CAD build for the part. Positions are in the model's coordinates, mm. Face numbers are marked on the shaded views. A direction names the side the tool comes from. Coordinates: 2 decimals unless noted, no trailing zeros. Order: outer loops, then holes, each group sorted by start corner. A loop starts at its lowest first (then second) coordinate and runs counter-clockwise, first axis right, second up. Notation, with made-up numbers: (68.25, -9.5) - (105.25, -9.5) arc R26 ccw to (105.25, 16.5) - close; hole circle Ø9 at (43.25, -5.5). An arc over 180 degrees is marked (long way). Return JSON: item names as keys, results as strings.
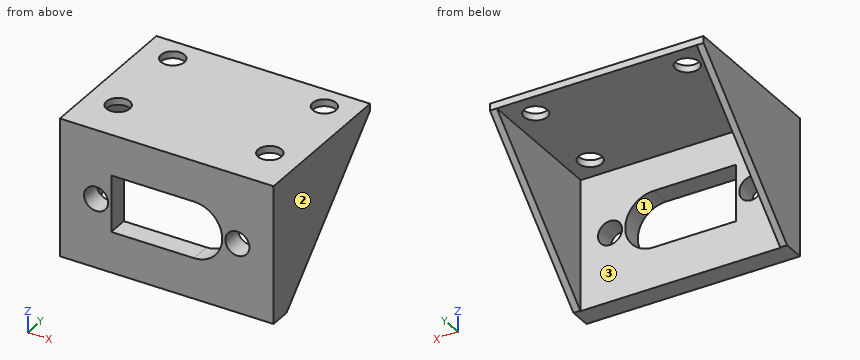
from build123d import *

# Parameters (mm, degrees)
SKETCH_W        = 31
SKETCH_H        = 20
SKETCH_R        = 1.75
PAD_DEPTH       = 3
PAD001_DEPTH    = 20
SKETCH002_R     = 1.7
HOLE_DEPTH      = 25
CHAMFER_1_SIZE2 = 19
CHAMFER_1_SIZE  = 19.9
CHAMFER_2_SIZE2 = 19
CHAMFER_2_SIZE  = 19.9


with BuildPart() as part:
    # Sketch → Pad (new body)
    with BuildSketch(Plane.XZ):
        with Locations((15.5, 10)):
            Rectangle(SKETCH_W, SKETCH_H)
        with Locations((25.75, 10)):
            Circle(SKETCH_R, mode=Mode.SUBTRACT)
        with Locations((5.25, 10)):
            Circle(SKETCH_R, mode=Mode.SUBTRACT)
        with BuildLine():
            ThreePointArc((19.45, 5.9), (23.55, 10), (19.45, 14.1))
            Line((19.45, 14.1), (7.45, 14.1))
            Line((7.45, 14.1), (7.45, 5.9))
            Line((7.45, 5.9), (19.45, 5.9))
        make_face(mode=Mode.SUBTRACT)
    extrude(amount=PAD_DEPTH)

    # Sketch001 (on Face11 of Pad) → Pad001 (join)
    with BuildSketch(Plane(origin=(0, 0, 0), x_dir=(1, 0, 0), z_dir=(0, 1, 0))):
        Polygon((31, 0), (31, -20), (0, -20), (0, 0), (1, 0), (1, -19), (30, -19), (30, 0), align=None)
    extrude(amount=PAD001_DEPTH)

    # Sketch002 (on Face13 of Pad001) → Hole (cut)
    with BuildSketch(Plane(origin=(0, 0, 19), x_dir=(1, 0, 0), z_dir=(0, 0, -1))):
        with Locations((4.5, -3.5)):
            Circle(SKETCH002_R)
        with Locations((26.5, -3.5)):
            Circle(SKETCH002_R)
        with Locations((26.5, -16.5)):
            Circle(SKETCH002_R)
        with Locations((4.5, -16.5)):
            Circle(SKETCH002_R)
    extrude(amount=-HOLE_DEPTH, mode=Mode.SUBTRACT)

    # Chamfer 1
    chamfer_1_edges = [part.edges().sort_by_distance(p)[0] for p in [
        (30.5, 20, 0),
    ]]
    chamfer_1_side = part.faces().sort_by_distance((30.5, 10, 0))[0]
    chamfer(chamfer_1_edges, length=CHAMFER_1_SIZE, length2=CHAMFER_1_SIZE2, reference=chamfer_1_side)

    # Chamfer 2
    chamfer_2_edges = [part.edges().sort_by_distance(p)[0] for p in [
        (0.5, 20, 0),
    ]]
    chamfer_2_side = part.faces().sort_by_distance((0.5, 10, 0))[0]
    chamfer(chamfer_2_edges, length=CHAMFER_2_SIZE, length2=CHAMFER_2_SIZE2, reference=chamfer_2_side)


solid = part.part
Item 1: Band-saw the part on A-A, the plane x = 4.5. List the corners of the cut face in (y, z).
Findings below:
{"outline": "(-3, 0) - (0, 0) - (0, 8.42) - (-3, 8.42) - close; (-3, 11.58) - (0, 11.58) - (0, 19) - (1.8, 19) - (1.8, 20) - (-3, 20) - close; (5.2, 19) - (14.8, 19) - (14.8, 20) - (5.2, 20) - close; (18.2, 19) - (20, 19) - (20, 20) - (18.2, 20) - close"}
Item 2: Which spindle directions (+Z, -Z, +X, -X, +Y, -Y) get a long thin tool onto all of the face, cutting with end or side? Do the marked faces 1, 2 and 3. Say none if no direction does.
Findings below:
{"face 1": "+Y, -Y", "face 2": "+Z, -Z, +X, +Y, -Y", "face 3": "-Z, +Y"}
Item 3: Drop flat-ended pins along their axis: P1, Ø5.5, axis at y = 7, z = 11, coming from the -X side; P2, Ø1, axis at x = 19.5, y = 7, coming from the -Z side; P3, Ø3, axis at x = 5.25, z = 10, coming from the -Y side; P4, Ø9.5, axis at x = 10, z = 5.5, coming from the +Y side. Give the stop position or say it passes through.
Findings below:
{"P1": "stops at x = 0", "P2": "stops at z = 19", "P3": "passes through", "P4": "stops at y = 0"}
Item 4: Wall check: L1, parallel to X at y = 3.5, z = 19.4; L2, parallel to Z at x = 5.25, y = -1.5; L3, parallel to X at y = 1.75, z = 7.5. Give the ranges that are in metal, low to high. Write a range as [from, to].
Findings below:
{"L1": "x = [0, 2.8], [6.2, 24.8], [28.2, 31]", "L2": "z = [0, 8.25], [11.75, 20]", "L3": "x = [0, 1], [30, 31]"}
Item 5: Band-saw the part on B-B, the plane x = 22. List the corners of the cut face in (y, z), then the cut area to 3 significant figures.
Findings below:
{"outline": "(-3, 0) - (0, 0) - (0, 6.79) - (-3, 6.79) - close; (-3, 13.21) - (0, 13.21) - (0, 19) - (20, 19) - (20, 20) - (-3, 20) - close", "area": "60.7 mm²"}
Item 6: Band-saw the part on C-C, the plane z = 8.75. Count the separate pieces of the cut face and the enclosed holes in it, then the cut area to 3 significant figures.
Findings below:
{"separate pieces": "4", "enclosed holes": "0", "area": "49.1 mm²"}
